Geometry: final body of the model. Coordinates: model frame, mm. Give positions to 0.01 mm unless a question says otherwise; leave off trailing zeros. Write each loop counter-clockwise with the first axis right and the second up, starting at its lowest first coordinate (ties: lowest second). Pieces come first, ordered by that corner, then holes. Notation, with made-up numbers: M 58,66 L 108,66 A27 cw 108,92 Z; hole C -30,2 d7. An arc over 180 degrees is marked long. Answer as a JSON object with one key per item and string values.
from build123d import *

# Parameters (mm, degrees)
F1_DEPTH = 10


with BuildPart() as f1:
    # F0 (on Top) → F1 (new body)
    with BuildSketch(Plane.XY):
        with BuildLine():
            ThreePointArc((-30.293809798, 5.9303317262), (-13.5387489786, -35.5502092603), (22.0330680191, -8.4206464354))
            ThreePointArc((22.0330680191, -8.4206464354), (21.1479502751, -1.419524921), (18.5482952641, 5.1410337217))
            ThreePointArc((18.5482952641, 5.1410337217), (10.523993366, 9.3012075006), (5.8590515306, 17.0429634058))
            ThreePointArc((5.8590515306, 17.0429634058), (-7.074281312, 19.6937803671), (-19.792655595, 16.1524692286))
            ThreePointArc((-19.792655595, 16.1524692286), (-23.8307305262, 9.7958026502), (-30.293809798, 5.9303317262))
        make_face()
        with BuildLine():
            ThreePointArc((5.8590515306, 17.0429634058), (10.523993366, 9.3012075006), (18.5482952641, 5.1410337217))
            ThreePointArc((18.5482952641, 5.1410337217), (13.146861043, 12.0975781831), (5.8590515306, 17.0429634058))
        make_face()
        with BuildLine():
            ThreePointArc((5.8590515306, 17.0429634058), (13.146861043, 12.0975781831), (18.5482952641, 5.1410337217))
            ThreePointArc((18.5482952641, 5.1410337217), (32.4160701368, 8.5391186206), (38.5428073237, 21.4358334092))
            ThreePointArc((38.5428073237, 21.4358334092), (19.6895316542, 37.9246568937), (5.8590515306, 17.0429634058))
        make_face()
        with BuildLine():
            ThreePointArc((-18.8964610276, 21.484998477), (-48.3679268886, 31.1266686737), (-30.293809798, 5.9303317262))
            ThreePointArc((-30.293809798, 5.9303317262), (-25.7205702793, 11.7372262186), (-19.792655595, 16.1524692286))
            ThreePointArc((-19.792655595, 16.1524692286), (-19.1220697647, 18.7813420229), (-18.8964610276, 21.484998477))
        make_face()
        with BuildLine():
            ThreePointArc((-19.792655595, 16.1524692286), (-25.7205702793, 11.7372262186), (-30.293809798, 5.9303317262))
            ThreePointArc((-30.293809798, 5.9303317262), (-23.8307305262, 9.7958026502), (-19.792655595, 16.1524692286))
        make_face()
    extrude(amount=F1_DEPTH)


solid = f1.part
1) Pull-direction query (Z, two-part tool) for faces 1 (the flat face through (-7, 1, 0)), 2 (the flat face through (-7, 1, 10)); classes: pulls with the +Z half, pulls with the -Z half, needs draft (parallel to the pull), parting line crosses it, or undercut.
Geometry check:
{"face 1": "pulls with the -Z half", "face 2": "pulls with the +Z half"}
2) Cut plane A-A on y = 31. Return loops of the section in (x, z).
Geometry check:
{"outline": "M -48.46,0 L -21.96,0 L -21.96,10 L -48.46,10 Z; M 8.29,0 L 35.52,0 L 35.52,10 L 8.29,10 Z"}
3) Cut plane B-B on z = 8.5. Return loops of the section in (x, y) (3 decimals), and give its area (3 significant figures).
Geometry check:
{"outline": "M -30.294,5.93 A28.131 ccw long 18.548,5.141 A16.637 ccw long 5.859,17.043 A28.131 ccw -19.793,16.152 A16.313 ccw long Z", "area": "4,120 mm2"}
4) Contact query for flat-ended pins moving along their axis: P1, Ø4, axis at x = -33, z = 2, coming from the +Y side; P2, Ø1.5, axis at x = 4.5, z = 6, coming from the -Y side; P3, Ø6, axis at x = -38.5, y = -0.5, coming from the +Z side; P4, Ø1.5, axis at y = -20.5, z = 8.5, coming from the -X side. Output: stop coordinate, or through.
Geometry check:
{"P1": "stops at y = 37.8", "P2": "stops at y = -34.77", "P3": "passes through", "P4": "stops at x = -31.85"}
5) Cut plane D-D on y = -3. Return loops of the section in (x, z).
Geometry check:
{"outline": "M -33.7,0 L 21.51,0 L 21.51,10 L -33.7,10 Z"}
6) Line query: line 1 (Y direction, x = -6, z = 7); line 2 (Y direction, x = 19, z = 8.5); line 3 (X direction, y = 30.5, z = 5.5). Output: solid intervals per line, ascending. Write a range as from..to.
Geometry check:
{"line 1": "y = -36.55..19.71", "line 2": "y = -21.13..4.29, 5.05..37.82", "line 3": "x = -48.8..-21.61, 7.95..35.86"}
7) Cut plane C-C on x = 23. Return loops of the section in (y, z), and give its area (3 significant figures).
Geometry check:
{"outline": "M 4.83,0 L 38.04,0 L 38.04,10 L 4.83,10 Z", "area": "332 mm2"}
